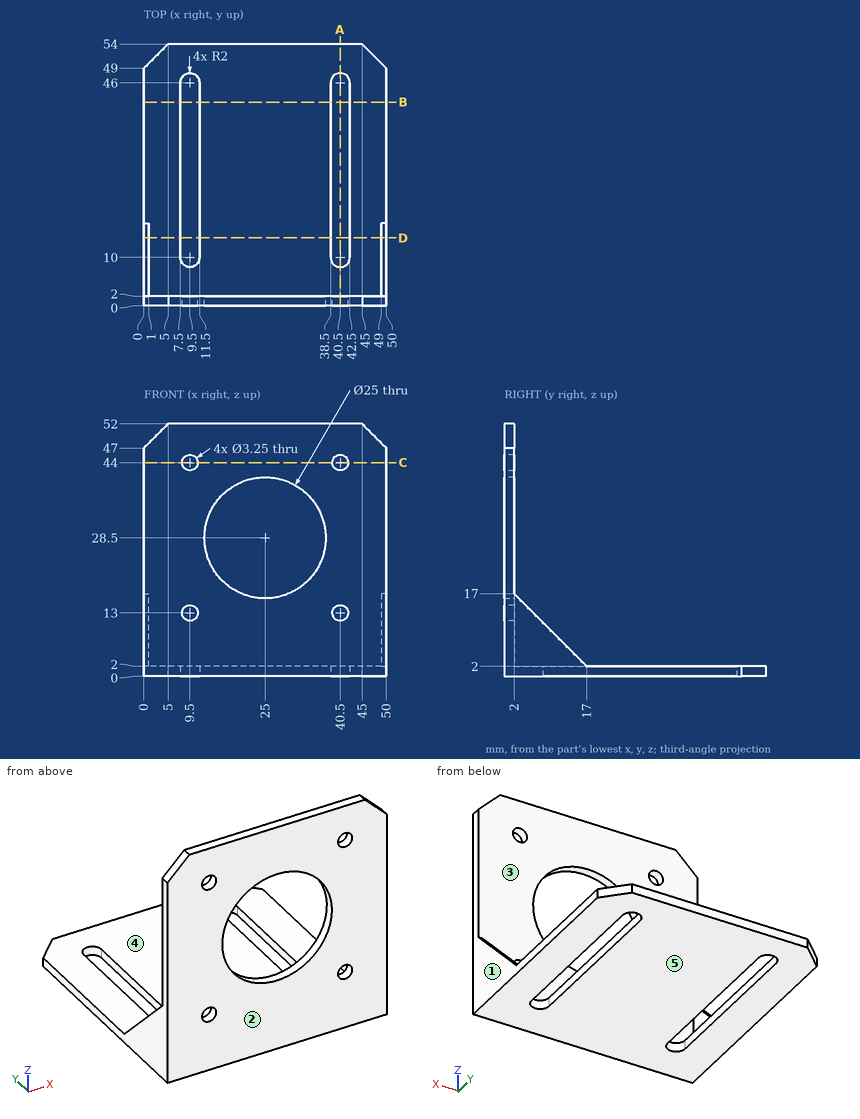
Study the drawing (mm; zero at the part's minimum x, y, z) and answer. A direction names the side the tool comes from. Give positions to 0.01 mm unless a question says otherwise; leave off trailing zeros. Write each loop counter-clockwise with the first axis right and the second up, starting at its lowest first coordinate (ties: lowest second). Pieces come first, ordered by that corner, then holes. Notation, with made-up numbers: (13, 68) -> (20, 68) arc R22 cw to (20, 107) -> close; hole circle Ø8 at (9.5, 86). An arc over 180 degrees is marked (long way). Write item = value, one per line.
Q1. Flat-ended cylindrical pins translate along their axes: pin 1 Ø3.5 at (x, z) = (40.5, 13) entering from +Y; pin 2 Ø10 at (x, y) = (43, 31.5) entering from +Z. Find the tip coordinate at first contact, or state that the pin passes through.
Computed values:
pin_1 = 2
pin_2 = 2
Q2. Section C-C on z = 44 is taken. Determine the outline of the cut face in (x, y) (3 decimals).
Computed values:
outline = (0, 0) -> (7.875, 0) -> (7.875, 2) -> (0, 2) -> close; (11.125, 0) -> (38.875, 0) -> (38.875, 2) -> (11.125, 2) -> close; (42.125, 0) -> (50, 0) -> (50, 2) -> (42.125, 2) -> close
Q3. For a pull along X with two mould halves and no side action, classify the marked faces 1, 2 and 3 as pulls with the +X half, pulls with the -X half, needs draft (parallel to the pull), parting line crosses it, or undercut.
Computed values:
face_1 = pulls with the +X half
face_2 = needs draft
face_3 = undercut
Q4. Section A-A on x = 40.5 is taken. Determine the outline of the cut face in (y, z) (3 decimals).
Computed values:
outline = (0, 0) -> (8, 0) -> (8, 2) -> (2, 2) -> (2, 11.375) -> (0, 11.375) -> close; (0, 14.625) -> (2, 14.625) -> (2, 42.375) -> (0, 42.375) -> close; (0, 45.625) -> (2, 45.625) -> (2, 52) -> (0, 52) -> close; (48, 0) -> (54, 0) -> (54, 2) -> (48, 2) -> close
Q5. Consider line 1 along Z through (x, y) = (40.5, 0.75) (3 decimals); line 2 along X through (y, z) = (1, 13) (3 decimals); line 3 along X through (y, z) = (1.35, 28.5). Determine where each line is inside the solid, lowest interval first.
Computed values:
line_1 = 0 to 11.375, 14.625 to 42.375, 45.625 to 52
line_2 = 0 to 7.875, 11.125 to 38.875, 42.125 to 50
line_3 = 0 to 12.5, 37.5 to 50
Q6. Section B-B on y = 42 is taken. Determine the outline of the cut face in (x, z).
Computed values:
outline = (0, 0) -> (7.5, 0) -> (7.5, 2) -> (0, 2) -> close; (11.5, 0) -> (38.5, 0) -> (38.5, 2) -> (11.5, 2) -> close; (42.5, 0) -> (50, 0) -> (50, 2) -> (42.5, 2) -> close
Q7. A tool of negligible diameter and unlimited length cuts with its end or side. For the marked faces 4 and 5, from which of +Z, -Z, +X, -X, +Y, -Y can it reach the whole face along a straight path? Write none if from no direction.
Computed values:
face_4 = +Z, +Y
face_5 = -Z, +X, -X, +Y, -Y
Q8. Section D-D on y = 14 is taken. Determine the outline of the cut face in (x, z).
Computed values:
outline = (0, 0) -> (7.5, 0) -> (7.5, 2) -> (1, 2) -> (1, 5) -> (0, 5) -> close; (11.5, 0) -> (38.5, 0) -> (38.5, 2) -> (11.5, 2) -> close; (42.5, 0) -> (50, 0) -> (50, 5) -> (49, 5) -> (49, 2) -> (42.5, 2) -> close
